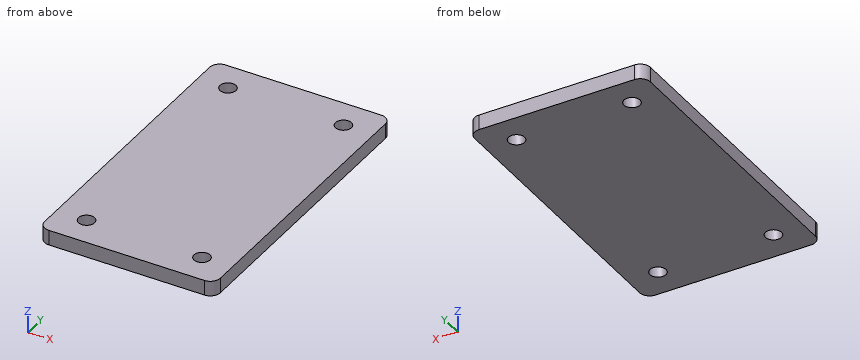
Autodesk Inventor part; units mm, degrees
ref_plane "YZ Plane" through (0, 0, 0) normal (1, 0, 0) x (0, 1, 0)
ref_plane "XZ Plane" through (0, 0, 0) normal (0, 1, 0) x (-1, 0, 0)
ref_plane "XY Plane" through (0, 0, 0) normal (0, 0, 1) x (1, 0, 0)
sketch "Skizze1" plane through (0, 0, 0) normal (0, 0, 1) x (1, 0, 0)
  line L0 (2, 0) -> (33, 0)
  line L1 (35, 2) -> (35, 58)
  line L2 (33, 60) -> (2, 60)
  line L3 (0, 58) -> (0, 2)
  arc A0 (2, 60) -> (0, 58) centre (2, 58) ccw
  arc A1 (0, 2) -> (2, 0) centre (2, 2) ccw
  arc A2 (33, 0) -> (35, 2) centre (33, 2) ccw
  arc A3 (35, 58) -> (33, 60) centre (33, 58) ccw
  circle A4 centre (6, 54) radius 1.6
  circle A5 centre (29, 54) radius 1.6
  circle A6 centre (6, 6) radius 1.6
  circle A7 centre (29, 6) radius 1.6
  point P0 (0, 0)
  dimension "d0" = 60
  dimension "d1" = 35
  dimension "d2" = 2
  dimension "d3" = 3.2
  dimension "d4" = 3.2
  dimension "d5" = 3.2
  dimension "d6" = 3.2
  dimension "d7" = 6
  dimension "d8" = 6
  dimension "d9" = 6
  dimension "d10" = 6
extrude "Extrusion1" add sketch "Skizze1" along normal blind 3
properties part number "103.017.01_Abdeckplatte_Extruderfuehrung" material "PMMA-Kunststoff"
Design review of the part built by this model. Coordinates are the model's own, in mm. Round coordinates to 2 decimals unless told otherwise and drop trailing zeros. Write each loop counter-clockwise with the first axis right and the second up, starting at its lowest first coordinate (ties: lowest second). Pieces come first, ordered by that corner, then holes.
Item 1: Wall thickness on L1, parallel to Y at x = 29, z = 2.3: over which ranges is the line inside the solid? List them lowest first.
Item 2: Consider section B-B on z = 0.85. Give the boundary of the cut face in (x, y).
Item 3: For pin 1 Ø2.5 at (x, y) = (29, 6) entering from +Z; pin 2 Ø5 at (x, y) = (6, 54) entering from -Z, all flat-tipped, find the tip position at first contact; note any pin that passes through.
Item 4: Consider section C-C on x = 29. Give the boundary of the cut face in (y, z).
Item 5: Consider section A-A on y = 54. Give the boundary of the cut face in (x, z).
Check values:
1. L1: y = 0 to 4.4, 7.6 to 52.4, 55.6 to 60
2. outline: (0, 2) arc R2 ccw to (2, 0) - (33, 0) arc R2 ccw to (35, 2) - (35, 58) arc R2 ccw to (33, 60) - (2, 60) arc R2 ccw to (0, 58) - close; hole circle Ø3.2 at (6, 6); hole circle Ø3.2 at (6, 54); hole circle Ø3.2 at (29, 6); hole circle Ø3.2 at (29, 54)
3. pin 1: passes through
3. pin 2: stops at z = 0
4. outline: (0, 0) - (4.4, 0) - (4.4, 3) - (0, 3) - close; (7.6, 0) - (52.4, 0) - (52.4, 3) - (7.6, 3) - close; (55.6, 0) - (60, 0) - (60, 3) - (55.6, 3) - close
5. outline: (0, 0) - (4.4, 0) - (4.4, 3) - (0, 3) - close; (7.6, 0) - (27.4, 0) - (27.4, 3) - (7.6, 3) - close; (30.6, 0) - (35, 0) - (35, 3) - (30.6, 3) - close
